Geometry: final body of the model. Coordinates: model frame, mm. A direction names the side the tool comes from. Round coordinates to 2 decimals unless told otherwise and drop trailing zeros. Loops run counter-clockwise (first coordinate to the right, second up) from the corner with the lowest first, then second, coordinate; pieces in that order, holes last. Notation, with made-up numbers: (74, -29) - (87, -29) arc R9 cw to (87, -21) - close; hole circle Ø3 at (58.5, 55.25). An arc over 180 degrees is marked (long way). Write item = value, one per line. Start each with the question number.
Item 1: First-contact query: pin 1 (4.5 mm diameter, centred on x = 0, y = -3.5, fed in from +Z); pin 2 (3 mm diameter, centred on x = -4.5, z = 63.5, fed in from +Y); pin 3 (1.5 mm diameter, centred on y = 3, z = 32, fed in from -X); pin 4 (5 mm diameter, centred on x = 0, y = 0, fed in from -Z). Flat tips, straight axial feed; report the tip coordinate or a pass-through.
Item 2: Draft query along Y for faces 1 (the conical face through (15.254, -3.387, 0.125)), 2 (the flat face through (-15.1, 8.85, 6.93)), 3 (the cylindrical face through (-0.07, -14.46, 8.62)), 4 (the flat face through (-10, -7, 80)). Return one class per face: pulls with the +Y half, pulls with the -Y half, needs draft (parallel to the pull), parting line crosses it, or undercut.
Item 3: Section A-A (z = 77). Return loops of the section in (x, y).
Item 4: Access query for faces 5 (the conical face through (-0.25, -10.695, 6.87)), 6 (the conical face through (-9.22, -5.42, 6.73)), 7 (the flat face through (-9.2, -15.4, 2)), 8 (the cylindrical face through (0.66, -14.985, 88.127)), 9 (the flat face through (9.583, 16.646, 7.07)). Directions: +Z, -Z, +X, -X, +Y, -Y. A direction counts if a zero-diameter tool reaches every point of the face in a straight line with its end or side. Return the directions, or none.
Item 5: Line query: line 1 (Y direction, x = 0, z = 58); line 2 (Z direction, x = 1, y = -14); line 3 (Y direction, x = 0, z = 2.25). Output: solid intervals per line, ascending. Write a range as from..to.
Autodesk Inventor part; units mm, degrees
ref_plane "Plan de construction1" through (0, 0, 2) normal (0, 0, -1) x (-1, 0, 0)
ref_plane "YZ Plane" through (0, 0, 0) normal (1, 0, 0) x (0, 1, 0)
ref_plane "XZ Plane" through (0, 0, 0) normal (0, 1, 0) x (-1, 0, 0)
sketch "Esquisse1" plane through (0, 0, 0) normal (1, 0, 0) x (0, 1, 0)
  line L0 (0, 0) -> (0, 68.1349)
  line L1 (15, 83.6949) -> (15, 12)
  line L2 (15.5, 0) -> (4, 0)
  line L3 (4, 0) -> (4, 4)
  line L4 (4, 4) -> (9.5, 4)
  line L5 (15, 90) -> (11, 90)
  line L6 (15, 12) -> (17.5, 12)
  line L7 (17.5, 12) -> (17.5, 2)
  line L8 (17.5, 2) -> (15.5, 0)
  line L9 (12.5, 12) -> (9.5, 9)
  line L10 (9.5, 9) -> (9.5, 4)
  line L11 (11, 90) -> (11, 80)
  line L12 (11, 80) -> (12.5, 80)
  line L13 (12.5, 80) -> (12.5, 12)
  line L14 (15, 90) -> (15, 86.3051)
  line L15 (15, 86.3051) -> (12.7, 87.1422)
  line L16 (12.7, 87.1422) -> (12.7, 82.8578)
  line L17 (12.7, 82.8578) -> (15, 83.6949)
  circle A0 centre (14.2, 85) radius 1.5 construction
  dimension "d1" = 30
  dimension "d2" = 8
  dimension "d3" = 4
  dimension "d5" = 2.5
  dimension "d6" = 2
  dimension "d7" = 2
  dimension "d8" = 10
  dimension "d26" = 3
  dimension "d27" = 3
  dimension "d31" = 2.5
  dimension "d32" = 4
  dimension "d34" = 10
  dimension "d35" = 78
  dimension "d36" = 70
  dimension "d37" = 70
  dimension "d38" = 3
  dimension "d39" = 0.8
  dimension "d40" = 5
revolve "Révolution1" add sketch "Esquisse1" angle 360 about axis through (0, 0, 0) along (0, 0, 1)
ref_plane "Plan de construction1" through (0, 0, 2) normal (0, 0, -1) x (-1, 0, 0)
sketch "Esquisse3" plane through (0, 0, 2) normal (0, 0, -1) x (-1, 0, 0)
  line L0 (10.1036, 17.5) -> (20.2073, 0)
  line L1 (20.2073, 0) -> (10.1036, -17.5)
  line L2 (10.1036, -17.5) -> (-10.1036, -17.5)
  line L3 (-10.1036, -17.5) -> (-20.2073, 0)
  line L4 (-20.2073, 0) -> (-10.1036, 17.5)
  line L5 (-10.1036, 17.5) -> (10.1036, 17.5)
  circle A0 centre (0, 0) radius 17.5
extrude "Extrusion1" add sketch "Esquisse3" against normal blind 10 contours L0 A0 L5 | L0 L1 A0 | A0 L4 L5 | A0 L3 L4 | L1 L2 A0 | A0 L2 L3
chamfer "Chanfrein1" distance 2 angle 45 1 edges at (0, -9.5, 4)
chamfer "Chanfrein2" distance 2 angle 45 6 edges at (10.1036, 17.5, 7) (-10.1036, 17.5, 7) (-20.2073, 0, 7) (-10.1036, -17.5, 7) (10.1036, -17.5, 7) (20.2073, 0, 7)
sketch "Esquisse4" plane through (-8.1036, -17.5, 2) normal (0, -1, 0) x (1, 0, 0)
  line L0 (16.2073, 10) -> (16.2073, 0)
  line L1 (0, 10) -> (16.2073, 10)
  line L2 (0, 0) -> (0, 10)
  line L3 (0, 0) -> (8.1036, 0)
  line L4 (8.1036, 0) -> (16.2073, 0)
  point P0 (8.1036, -2)
  point P1 (8.1036, 5)
  point P2 (16.2073, 5)
hole "Perçage1" at (0, -17.5, 7) direction (0, 1, 0) diameter 3.242 depth 6 tip angle 118
chamfer "Chanfrein3" distance 1 angle 45 2 edges at (0, -11, 90) (0, -11, 80)
pattern_circular "Réseau circulaire1" count 3 over 120 about axis through (0, 0, -10) along (0, 0, 1) of "Perçage1" both ways yes
equation "\"d7\" = d6"
equation "\"d27\" = d26"
equation "\"d37\" = d36"
properties part number "piston_reservoir" material "Acier, galvanisé"
Taken from the geometry:
q1.pin_1 = 4
q1.pin_2 = 14.7
q1.pin_3 = -14.83
q1.pin_4 = through
q2.face_1 = parting line crosses it
q2.face_2 = pulls with the +Y half
q2.face_3 = needs draft
q2.face_4 = undercut
q3.outline = circle Ø30 at (0, 0); hole circle Ø25 at (0, 0)
q4.face_5 = -Y
q4.face_6 = none
q4.face_7 = -Z, -X, -Y
q4.face_8 = +Z
q4.face_9 = +Z, -Z, +X, +Y
q5.line_1 = -15..-12.5, 12.5..15
q5.line_2 = 0..5.72, 8.28..83.34, 86.66..90
q5.line_3 = -17.5..-4, 4..17.5
